Part model, mm, in its own coordinate system. A direction names the side the tool comes from. Coordinates: 2 decimals unless noted, no trailing zeros. Order: outer loops, then holes, each group sorted by start corner. A loop starts at its lowest first (then second) coordinate and runs counter-clockwise, first axis right, second up.
```python
from build123d import *

# Parameters (mm, degrees)
BOSS_EXTRUDE1_DEPTH = 3.175
SKETCH2_W           = 107.95
SKETCH2_H           = 3.175
CUT_EXTRUDE1_DEPTH  = 355.989990176
SKETCH3_R           = 1.5875
CUT_EXTRUDE2_DEPTH  = 355.989990176
SKETCH4_W           = 34.925
SKETCH4_H           = 152.4
CUT_EXTRUDE3_DEPTH  = 355.989990176
FILLET1_R           = 1.5875


with BuildPart() as part:
    # Sketch1 → Boss-Extrude1 (new body)
    with BuildSketch(Plane(origin=(0, 0, 0), x_dir=(1, 0, 0), z_dir=(0, 1, 0))):
        Polygon((130.175, 0), (158.75, 0), (158.75, 317.5), (0, 317.5), (0, 0), (28.575, 0), (28.575, -3.175), (130.175, -3.175), align=None)
    extrude(amount=BOSS_EXTRUDE1_DEPTH)

    # Sketch2 → Cut-Extrude1 (cut, through all)
    with BuildSketch(Plane(origin=(0, 3.175, 0), x_dir=(1, 0, 0), z_dir=(0, 1, 0))):
        with Locations((79.375, 315.9125)):
            Rectangle(SKETCH2_W, SKETCH2_H)
    extrude(amount=-CUT_EXTRUDE1_DEPTH, mode=Mode.SUBTRACT)

    # Sketch3 → Cut-Extrude2 (cut, through all)
    with BuildSketch(Plane(origin=(0, 3.175, 0), x_dir=(1, 0, 0), z_dir=(0, 1, 0))):
        with Locations(Location((12.7, 6.35, 0), (0, 0, 270))):
            Circle(SKETCH3_R)
        with Locations(Location((149.225, 6.35, 0), (0, 0, 270))):
            Circle(SKETCH3_R)
        with Locations(Location((149.225, 69.85, 0), (0, 0, 270))):
            Circle(SKETCH3_R)
        with Locations(Location((36.5125, 79.375, 0), (0, 0, 270))):
            Circle(SKETCH3_R)
        Polygon((21.680256121, 6.35), (12.7, 15.330256121), (12.7, 66.675), (19.05, 73.025), (39.142756121, 73.025), (45.492756121, 79.375), (130.719743879, 79.375), (149.225, 60.869743879), (149.225, 15.330256121), (140.244743879, 6.35), align=None)
    extrude(amount=-CUT_EXTRUDE2_DEPTH, mode=Mode.SUBTRACT)

    # Sketch4 → Cut-Extrude3 (cut, through all)
    with BuildSketch(Plane(origin=(0, 3.175, 0), x_dir=(1, 0, 0), z_dir=(0, 1, 0))):
        with Locations((30.1625, 225.425)):
            Rectangle(SKETCH4_W, SKETCH4_H)
    extrude(amount=-CUT_EXTRUDE3_DEPTH, mode=Mode.SUBTRACT)

    # Fillet1
    fillet1_edges = [part.edges().sort_by_distance(p)[0] for p in [
        (25.4, 1.5875, -314.325),
        (25.4, 1.5875, -317.5),
        (0, 1.5875, -317.5),
        (0, 1.5875, 0),
        (28.575, 1.5875, 0),
        (28.575, 1.5875, 3.175),
        (130.175, 1.5875, 3.175),
        (130.175, 1.5875, 0),
        (158.75, 1.5875, 0),
        (158.75, 1.5875, -317.5),
        (133.35, 1.5875, -317.5),
        (133.35, 1.5875, -314.325),
        (140.244743879, 1.5875, -6.35),
        (149.225, 1.5875, -15.330256121),
        (149.225, 1.5875, -60.869743879),
        (130.719743879, 1.5875, -79.375),
        (45.492756121, 1.5875, -79.375),
        (39.142756121, 1.5875, -73.025),
        (19.05, 1.5875, -73.025),
        (12.7, 1.5875, -66.675),
        (21.680256121, 1.5875, -6.35),
        (12.7, 1.5875, -15.330256121),
        (12.7, 1.5875, -149.225),
        (47.625, 1.5875, -149.225),
        (12.7, 1.5875, -301.625),
        (47.625, 1.5875, -301.625),
    ]]
    fillet(fillet1_edges, radius=FILLET1_R - 0.0001)  # a hair under: the kernel refuses the full size


solid = part.part
```
(1) Tool access for faces 3 (the face through (139.849, 1.61, -70.245)), 4 (the face through (78, 0, -195)): list every direction of +Z, -Z, +X, -X, +Y, -Y with a clear straight run to the whole face (end or side of a thin tool).
(2) Drop a flat-ended pin along its axis: pin 1 (1 mm diameter, centred on x = 138.5, y = 2, fed in from +Z). Give the stop position or say it passes through.
(3) Probe line 1 (Z direction, x = 22.5, y = 0.25) (3 decimals); line 2 (Z direction, x = 118, y = 2.2) (3 decimals); line 3 (Z direction, x = 29.5, y = 2.4) (3 decimals). List the from-to ranges inside material, lowest first.
(4) Slice it at A-A, the plane x = 122.5. Give the cut face in (y, z) (3 decimals).
(5) Slice it at B-B, the plane y = 2.15. State how many separate pieces and enclosed holes the cut face has, then the cut area to 3 significant figures.
(6) Pull direction Z, two halves, no side cores. Call faces 1 (the face through (42.28, 1.61, -76.16)), 2 (the face through (78, 3.175, -195)): +Z half, -Z half, draft (parallel to the pull), parting line (faces both ways), or undercut.
Here are the results:
1. face 3: +Y, -Y
1. face 4: +Z, -Z, +X, -X, -Y
2. pin 1: stops at z = 0
3. line 1: z = -317.5 to -301.625, -149.225 to -73.025, -6.35 to 0
3. line 2: z = -314.325 to -79.375, -6.35 to 3.175
3. line 3: z = -314.325 to -301.625, -149.225 to -73.025, -6.35 to 3.03
4. outline: (0, -314.325) - (3.175, -314.325) - (3.175, -79.375) - (0, -79.375) - close; (0, -6.35) - (3.175, -6.35) - (3.175, 3.175) - (0, 3.175) - close
5. separate pieces: 1
5. enclosed holes: 6
5. area: 35,500 mm2
6. face 1: undercut
6. face 2: draft
